The drawing under review shows one solid part. Ordinate dimensions are in mm from its lowest x, y, z. Coordinates: 2 decimals unless noted, no trailing zeros. Order: outer loops, then holes, each group sorted by start corner. A loop starts at its lowest first (then second) coordinate and runs counter-clockwise, first axis right, second up. Notation, with made-up numbers: (41.25, -26) -> (99.25, -26) arc R33 cw to (99.25, 11) -> close; hole circle Ø10 at (69, 24.25). An arc over 180 degrees is marked (long way). Write item = value, one per line.
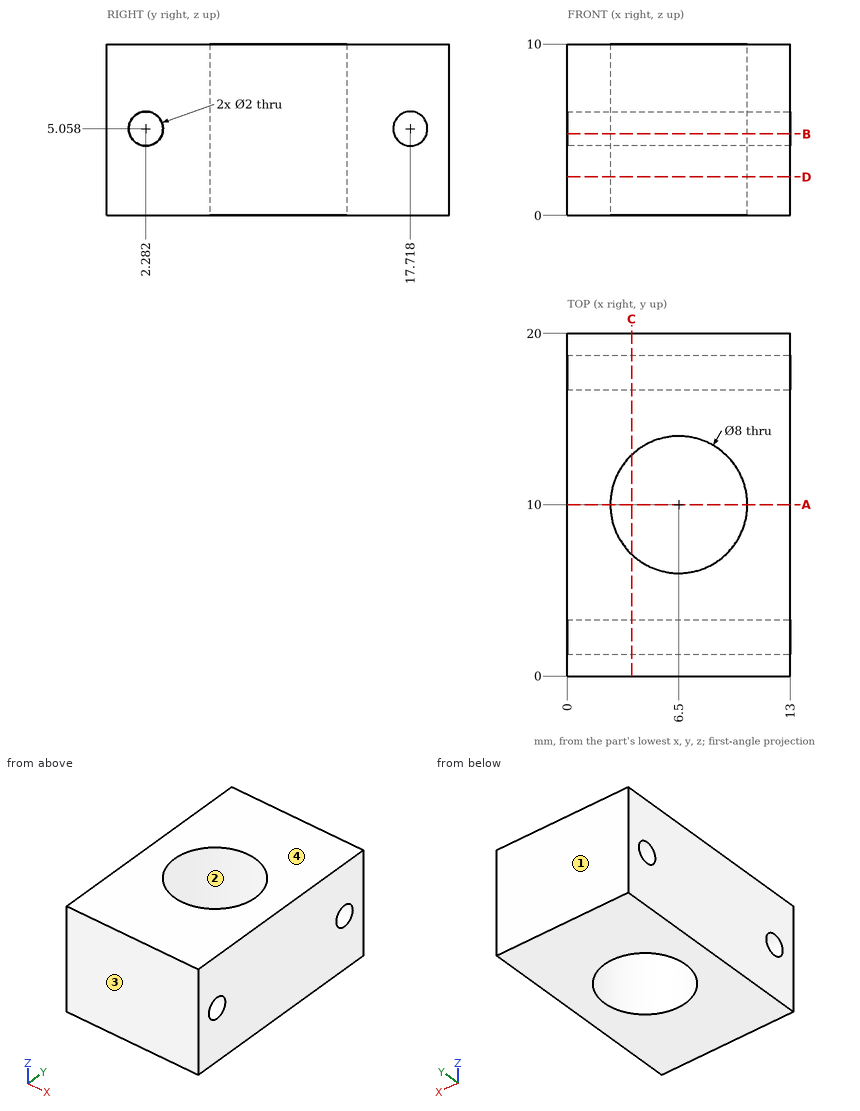
(1) We need section D-D (z = 2.25). Write out the cut boundary in (x, y).
Report:
outline = (0, 0) -> (13, 0) -> (13, 20) -> (0, 20) -> close; hole circle Ø8 at (6.5, 10)
(2) We need section C-C (x = 3.75). Write out the cut boundary in (y, z) (1 decimal), and give its area (3 significant figures).
Report:
outline = (0, 0) -> (7.1, 0) -> (7.1, 10) -> (0, 10) -> close; (12.9, 0) -> (20, 0) -> (20, 10) -> (12.9, 10) -> close; hole circle Ø2 at (2.3, 5.1); hole circle Ø2 at (17.7, 5.1)
area = 136 mm²
(3) For L1, parallel to Y at x = 2, z = 5.5 (1 decimal); L2, parallel to Y at x = 6.5, z = 4.25 (1 decimal); L3, parallel to Y at x = 5.5, z = 4.25 (1 decimal), list the stretches that pass through material, from the lowest coordinate up.
Report:
L1 = 0 to 1.4, 3.2 to 16.8, 18.6 to 20
L2 = 0 to 1.7, 2.9 to 6, 14 to 17.1, 18.3 to 20
L3 = 0 to 1.7, 2.9 to 6.1, 13.9 to 17.1, 18.3 to 20
(4) The part is to be moulded in two halves that separate along Y. For the marked faces 1, 2, 3 and 4, say which applies: released by +Y, released by -Y, zero draft, split by the parting line, or undercut.
Report:
face_1 = released by +Y
face_2 = undercut
face_3 = released by -Y
face_4 = zero draft
(5) We need section B-B (z = 4.75). Write out the cut boundary in (x, y).
Report:
outline = (0, 0) -> (13, 0) -> (13, 1.33) -> (0, 1.33) -> close; (0, 3.23) -> (13, 3.23) -> (13, 16.77) -> (0, 16.77) -> close; (0, 18.67) -> (13, 18.67) -> (13, 20) -> (0, 20) -> close; hole circle Ø8 at (6.5, 10)
(6) We need section A-A (y = 10). Write out the cut boundary in (x, z).
Report:
outline = (0, 0) -> (2.5, 0) -> (2.5, 10) -> (0, 10) -> close; (10.5, 0) -> (13, 0) -> (13, 10) -> (10.5, 10) -> close
